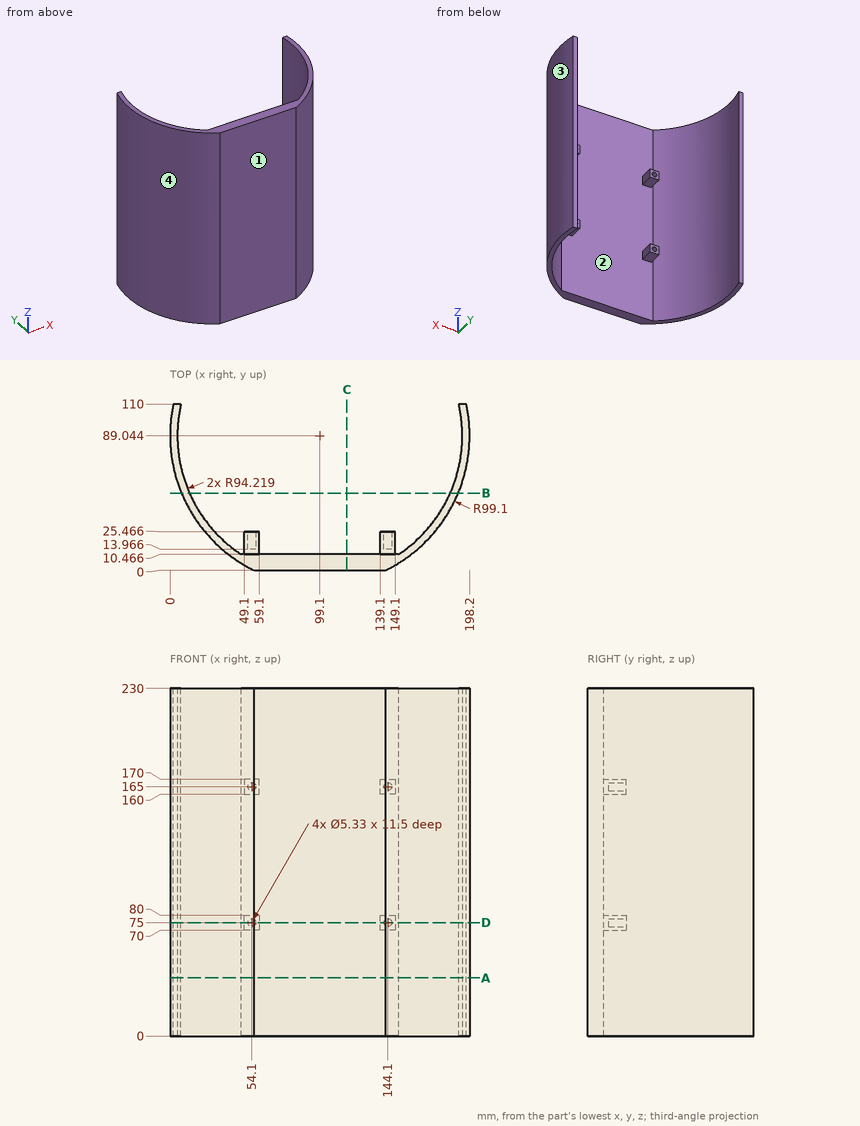
For this review, use the dimensioned drawing (mm, ordinates from the lowest corner) and the shaded views. Coordinates: 2 decimals unless noted, no trailing zeros. Loops run counter-clockwise (first coordinate to the right, second up) from the corner with the lowest first, then second, coordinate; pieces in that order, holes last. Notation, with made-up numbers: (-22, 87.5) -> (-13, 87.5) arc R32 cw to (-13, 115.5) -> close; hole circle Ø5 at (-7, 42). An arc over 180 degrees is marked (long way). Use a Markdown table: item, result. Add a question column.
1. Add section B-B on y = 51. Write out the cut boundary in (x, z).
2. Clearance check with flat-ended pins moving along their axes: pin 1 Ø10 at (y, z) = (31.5, 160.5) entering from -X; pin 2 Ø3 at (x, y) = (144.5, 18.5) entering from +Z; pin 3 Ø10 at (y, z) = (59.5, 138.5) entering from +X. State where each tip first meets the part, or that it passes through.
3. Draft analysis for pull direction X (two halves, no side actions). For the marked faces 1, 2, 3 and 4, state which applies: pulls with the +X half, pulls with the -X half, needs draft (parallel to the pull), parting line crosses it, or undercut.
4. Add section C-C on x = 117. Write out the cut boundary in (y, z).
5. Add section D-D on z = 75. Write out the cut boundary in (x, y) (1 decimal).
6. Add section A-A on z = 38.5. Write out the cut boundary in (x, y), plus the area to 3 significant figures.
7. To check wall thickness, follow line 1 (X direction, y = 88, z = 148); line 2 (X direction, y = 21.25, z = 165) (1 decimal); line 3 (X direction, y = 20.75, z = 165) (1 decimal). State the ranges of each line that lie inside material, in increasing order.
Returned:
| question | item | result |
|---|---|---|
| 1 | outline | (7.59, 0) -> (12.9, 0) -> (12.9, 230) -> (7.59, 230) -> close; (185.3, 0) -> (190.61, 0) -> (190.61, 230) -> (185.3, 230) -> close |
| 2 | pin 1 | stops at x = 15.08 |
| 2 | pin 2 | stops at z = 170 |
| 2 | pin 3 | stops at x = 195.11 |
| 3 | face 1 | needs draft |
| 3 | face 2 | undercut |
| 3 | face 3 | pulls with the +X half |
| 3 | face 4 | pulls with the -X half |
| 4 | outline | (0, 0) -> (10.47, 0) -> (10.47, 230) -> (0, 230) -> close |
| 5 | outline | (2.2, 110) arc R99.1 ccw to (55.6, 0) -> (142.6, 0) arc R99.1 ccw to (196, 110) -> (191, 110) arc R94.2 cw to (151.1, 10.5) -> (149.1, 10.5) -> (149.1, 25.5) -> (146.8, 25.5) -> (146.8, 14) -> (141.4, 14) -> (141.4, 25.5) -> (139.1, 25.5) -> (139.1, 10.5) -> (59.1, 10.5) -> (59.1, 25.5) -> (56.8, 25.5) -> (56.8, 14) -> (51.4, 14) -> (51.4, 25.5) -> (49.1, 25.5) -> (49.1, 10.5) -> (47.1, 10.5) arc R94.2 cw to (7.2, 110) -> close |
| 6 | outline | (2.24, 110) arc R99.1 ccw to (55.6, 0) -> (142.6, 0) arc R99.1 ccw to (195.96, 110) -> (190.96, 110) arc R94.22 cw to (151.09, 10.47) -> (47.11, 10.47) arc R94.22 cw to (7.24, 110) -> close |
| 6 | area | 2,200 mm² |
| 7 | line 1 | x = 0.01 to 4.89, 193.31 to 198.19 |
| 7 | line 2 | x = 26.8 to 33.7, 49.1 to 51.4, 56.8 to 59.1, 139.1 to 141.4, 146.8 to 149.1, 164.5 to 171.4 |
| 7 | line 3 | x = 27.3 to 34.2, 49.1 to 51.4, 56.8 to 59.1, 139.1 to 141.4, 146.8 to 149.1, 164 to 170.9 |
